```python
from build123d import *

# Parameters (mm, degrees)
F0_W         = 63
F0_H         = 137
F0_W_2       = 57
F0_H_2       = 131
F1_DEPTH     = 2
F4_DEPTH     = 36
F5_T4_DEPTH  = 38
F5_T10_DEPTH = 38
F5_T17_DEPTH = 38
F5_T23_DEPTH = 38
F5_T30_DEPTH = 38
F5_T36_DEPTH = 38
F5_T43_DEPTH = 38
F5_T49_DEPTH = 38
F6_R         = 2


# Not quite as in the source:
# - a fillet or chamfer that OpenCascade refuses, or shapes differently, is made with other operations: its cross-section is extruded or revolved along the edge and cut away or added


with BuildPart() as f1:
    # F0 (on Top) → F1 (new body)
    with BuildSketch(Plane.XY):
        Rectangle(F0_W, F0_H)
        Rectangle(F0_W_2, F0_H_2, mode=Mode.SUBTRACT)
    extrude(amount=F1_DEPTH)

    # F3 (on face) → F4 (join, through all)
    with BuildSketch(Plane.XY.offset(2)):
        Polygon((-26.5, 68.5), (-31.5, 68.5), (-31.5, 63.5), (-28.5, 63.5), (-28.5, 65.5), (-26.5, 65.5), align=None)
        Polygon((31.5, 68.5), (26.5, 68.5), (26.5, 65.5), (28.5, 65.5), (28.5, 63.5), (31.5, 63.5), align=None)
    extrude(amount=F4_DEPTH)

    # F5: fillet of radius 3 on 2 edges, made by hand


with BuildPart() as f5_tool2:
    # F5_s3 → F5_t4 (new body)
    with BuildSketch(Plane.XY):
        with BuildLine():
            ThreePointArc((-25.5, 65.5), (-27.6213203436, 64.6213203436), (-28.5, 62.5))
            Line((-28.5, 62.5), (-28.5, 65.5))
            Line((-28.5, 65.5), (-25.5, 65.5))
        make_face()
    extrude(amount=F5_T4_DEPTH)

    split(bisect_by=Plane.XY.offset(2), keep=Keep.BOTTOM)

    split(bisect_by=Plane.YZ.offset(-26.5), keep=Keep.TOP)


with BuildPart() as f1_1:
    add(f1.part)

    # F5_t1: union F5_tool2
    add(f5_tool2.part)


with BuildPart() as f5_tool8:
    # F5_s9 → F5_t10 (new body)
    with BuildSketch(Plane.XY):
        with BuildLine():
            ThreePointArc((-25.5, 65.5), (-27.6213203436, 64.6213203436), (-28.5, 62.5))
            Line((-28.5, 62.5), (-28.5, 65.5))
            Line((-28.5, 65.5), (-25.5, 65.5))
        make_face()
    extrude(amount=F5_T10_DEPTH)

    split(bisect_by=Plane.XY.offset(2), keep=Keep.BOTTOM)

    split(bisect_by=Plane.XZ.offset(-63.5), keep=Keep.BOTTOM)

    split(bisect_by=Plane.YZ.offset(-26.5), keep=Keep.BOTTOM)


with BuildPart() as f1_2:
    add(f1_1.part)

    # F5_t7: union F5_tool8
    add(f5_tool8.part)


with BuildPart() as f5_tool15:
    # F5_s16 → F5_t17 (new body)
    with BuildSketch(Plane.XY):
        with BuildLine():
            ThreePointArc((-25.5, 65.5), (-27.6213203436, 64.6213203436), (-28.5, 62.5))
            Line((-28.5, 62.5), (-28.5, 65.5))
            Line((-28.5, 65.5), (-25.5, 65.5))
        make_face()
    extrude(amount=F5_T17_DEPTH)

    split(bisect_by=Plane.XY.offset(2), keep=Keep.BOTTOM)

    split(bisect_by=Plane.XZ.offset(-63.5), keep=Keep.TOP)


with BuildPart() as f1_3:
    add(f1_2.part)

    # F5_t14: union F5_tool15
    add(f5_tool15.part)


with BuildPart() as f5_tool21:
    # F5_s22 → F5_t23 (new body)
    with BuildSketch(Plane.XY):
        with BuildLine():
            ThreePointArc((-25.5, 65.5), (-27.6213203436, 64.6213203436), (-28.5, 62.5))
            Line((-28.5, 62.5), (-28.5, 65.5))
            Line((-28.5, 65.5), (-25.5, 65.5))
        make_face()
    extrude(amount=F5_T23_DEPTH)

    split(bisect_by=Plane.XY.offset(2), keep=Keep.TOP)

    split(bisect_by=Plane.XZ.offset(-63.5), keep=Keep.BOTTOM)

    split(bisect_by=Plane.YZ.offset(-26.5), keep=Keep.BOTTOM)


with BuildPart() as f1_4:
    add(f1_3.part)

    # F5_t20: union F5_tool21
    add(f5_tool21.part)


with BuildPart() as f5_tool28:
    # F5_s29 → F5_t30 (new body)
    with BuildSketch(Plane.XY):
        with BuildLine():
            ThreePointArc((28.5, 62.5), (27.6213203436, 64.6213203436), (25.5, 65.5))
            Line((25.5, 65.5), (28.5, 65.5))
            Line((28.5, 65.5), (28.5, 62.5))
        make_face()
    extrude(amount=F5_T30_DEPTH)

    split(bisect_by=Plane.XY.offset(2), keep=Keep.BOTTOM)

    split(bisect_by=Plane.XZ.offset(-63.5), keep=Keep.TOP)


with BuildPart() as f1_5:
    add(f1_4.part)

    # F5_t27: union F5_tool28
    add(f5_tool28.part)


with BuildPart() as f5_tool34:
    # F5_s35 → F5_t36 (new body)
    with BuildSketch(Plane.XY):
        with BuildLine():
            ThreePointArc((28.5, 62.5), (27.6213203436, 64.6213203436), (25.5, 65.5))
            Line((25.5, 65.5), (28.5, 65.5))
            Line((28.5, 65.5), (28.5, 62.5))
        make_face()
    extrude(amount=F5_T36_DEPTH)

    split(bisect_by=Plane.XY.offset(2), keep=Keep.BOTTOM)

    split(bisect_by=Plane.XZ.offset(-63.5), keep=Keep.BOTTOM)

    split(bisect_by=Plane.YZ.offset(26.5), keep=Keep.TOP)


with BuildPart() as f1_6:
    add(f1_5.part)

    # F5_t33: union F5_tool34
    add(f5_tool34.part)


with BuildPart() as f5_tool41:
    # F5_s42 → F5_t43 (new body)
    with BuildSketch(Plane.XY):
        with BuildLine():
            ThreePointArc((28.5, 62.5), (27.6213203436, 64.6213203436), (25.5, 65.5))
            Line((25.5, 65.5), (28.5, 65.5))
            Line((28.5, 65.5), (28.5, 62.5))
        make_face()
    extrude(amount=F5_T43_DEPTH)

    split(bisect_by=Plane.XY.offset(2), keep=Keep.BOTTOM)

    split(bisect_by=Plane.YZ.offset(26.5), keep=Keep.BOTTOM)


with BuildPart() as f1_7:
    add(f1_6.part)

    # F5_t40: union F5_tool41
    add(f5_tool41.part)


with BuildPart() as f5_tool47:
    # F5_s48 → F5_t49 (new body)
    with BuildSketch(Plane.XY):
        with BuildLine():
            ThreePointArc((28.5, 62.5), (27.6213203436, 64.6213203436), (25.5, 65.5))
            Line((25.5, 65.5), (28.5, 65.5))
            Line((28.5, 65.5), (28.5, 62.5))
        make_face()
    extrude(amount=F5_T49_DEPTH)

    split(bisect_by=Plane.XY.offset(2), keep=Keep.TOP)

    split(bisect_by=Plane.XZ.offset(-63.5), keep=Keep.BOTTOM)

    split(bisect_by=Plane.YZ.offset(26.5), keep=Keep.TOP)


with BuildPart() as f1_8:
    add(f1_7.part)

    # F5_t46: union F5_tool47
    add(f5_tool47.part)

    # F6
    f6_edges = [f1_8.edges().sort_by_distance(p)[0] for p in [
        (-31.5, 68.5, 19),
        (31.5, 68.5, 19),
        (31.5, -68.5, 1),
        (-31.5, -68.5, 1),
        (28.5, -65.5, 1),
        (-28.5, -65.5, 1),
    ]]
    fillet(f6_edges, radius=F6_R)


solid = f1_8.part
```
Geometry: final body of the model. Coordinates: model frame, mm. A direction names the side the tool comes from. Coordinates: 2 decimals unless noted, no trailing zeros. Order: outer loops, then holes, each group sorted by start corner. A loop starts at its lowest first (then second) coordinate and runs counter-clockwise, first axis right, second up. Notation, with made-up numbers: M -15.5,80.5 L -6.5,80.5 A29 cw -6.5,116.5 Z; hole C 86.5,57.5 d7. An arc over 180 degrees is marked long. Answer in a Markdown table with one row per item. Add a question column.
Q1. Section query A-A on y = 7.5. Return the cut outline in (x, z), and give its area (3 significant figures).
Q2. Section query B-B on z = 30. Return the cut outline in (x, y), and give its area (3 significant figures).
Q3. Mould query, pull axis X, two halves, no side actions, for faces 6 (the flat face through (26.5, 67, 20)), 7 (the flat face through (31.5, 29, 1)), 8 (the flat face through (30, 0, 0)). Classes: released by +X, released by -X, zero draft, split by the parting line, or undercut.
Q4. Section query C-C on x = 6. Return the cut outline in (y, z).
Q5. Reachability of faces 1 (the flat face through (0, 68.5, 1)), 2 (the flat face through (-29, 66, 38)), 3 (the flat face through (-26.5, 67, 20)), 4 (the flat face through (30, 63.5, 20)), 5 (the cylindrical face through (27.64, 64.6, 18.73)) from +Z, -Z, +X, -X, +Y, -Y: full face, straight path, thin tool, end or side. Return the list, or none.
Q6. Contact query for flat-ended pins moving along their axis: P1, Ø1, axis at x = 2, y = 67, coming from the +Z side; P2, Ø1, axis at x = 30, z = 20, coming from the -Y side. Output: stop coordinate, or through.
Completed:
| question | item | result |
|---|---|---|
| 1 | outline | M -31.5,0 L -28.5,0 L -28.5,2 L -31.5,2 Z; M 28.5,0 L 31.5,0 L 31.5,2 L 28.5,2 Z |
| 1 | area | 12.0 mm2 |
| 2 | outline | M -31.5,63.5 L -28.33,63.5 A3 cw -26.5,65.33 L -26.5,68.5 L -29.5,68.5 A2 ccw -31.5,66.5 Z; M 26.5,65.33 A3 cw 28.33,63.5 L 31.5,63.5 L 31.5,66.5 A2 ccw 29.5,68.5 L 26.5,68.5 Z |
| 2 | area | 43.9 mm2 |
| 3 | face 6 | undercut |
| 3 | face 7 | released by +X |
| 3 | face 8 | zero draft |
| 4 | outline | M -68.5,0 L -65.5,0 L -65.5,2 L -68.5,2 Z; M 65.5,0 L 68.5,0 L 68.5,2 L 65.5,2 Z |
| 5 | face 1 | +Z, -Z, +X, -X, +Y |
| 5 | face 2 | +Z, +X, -X, +Y, -Y |
| 5 | face 3 | +Z, +Y, -Y |
| 5 | face 4 | +Z, +X, -X, -Y |
| 5 | face 5 | +Z, -Z |
| 6 | P1 | stops at z = 2 |
| 6 | P2 | stops at y = 63.5 |
